Read the model definition and answer for the solid it produces. Units are mm, in the model's axes. A direction names the side the tool comes from. Round coordinates to 2 decimals unless told otherwise and drop trailing zeros. Write each loop counter-clockwise with the first axis right and the second up, starting at its lowest first coordinate (ties: lowest second). Pieces come first, ordered by that corner, then holes. Notation, with made-up numbers: (31.25, 35) - (79.25, 35) arc R16 ccw to (79.25, 66) - close; hole circle Ø11 at (59, 12.5). An arc over 180 degrees is marked (long way). Answer as CSV lines item,"result". Start each with the question number.
1) Consider line 1 along X through (y, z) = (11.5, 0); line 2 along X through (y, z) = (19, -8.5); line 3 along Z through (x, y) = (11.5, 35.5). Determine where each line is inside the solid, lowest interval first.
2) For a pull along Y with two mould halves and no side action, classify faces 1 (the cylindrical face through (19.54, 4.55, -19.7)), 2 (the cylindrical face through (15.747, 2.986, 8.191)), 3 (the flat face through (6.3, 0, 16)) as +Y half, -Y half, draft (parallel to the pull), parting line (faces both ways), or undercut.
3) Find section D-D on y = 19. Determine the outline of the cut face in (x, z).
4) Find section C-C on y = 3. Determine the outline of the cut face in (x, z), then the cut area to 3 significant figures.
5) Which of the six approach directions +Z, -Z, +X, -X, +Y, -Y give full straight-line access (tool end or side, diameter ignored) to faces 4 (the flat face through (0, 5, -23.5)), 5 (the cylindrical face through (-14.531, 0.507, -15.846)), 6 (the cylindrical face through (19.524, 24.224, -4.336))?
6) Each of these flat-tipped pins is pushed along its axis until it touches: pin 1 (10 mm diameter, centred on x = 1, y = 17.5, fed in from +Z); pin 2 (9 mm diameter, centred on x = 17.68, z = 17.68, fed in from +Y); pin 3 (12 mm diameter, centred on x = 10.5, y = 24, fed in from +Z). Where does it stop, or does it pass through?
from build123d import *

# Parameters (mm, degrees)
SKETCH_4_R           = 2.75
CUT_EXTRUDE_1_DEPTH  = 54.141321022
SKETCH_5_OUTSIDE_W   = 80.762
SKETCH_5_OUTSIDE_H   = 80.762
SKETCH_5_OUTSIDE_W_2 = 47
SKETCH_5_OUTSIDE_H_2 = 47
CUT_EXTRUDE_2_DEPTH  = 54.141321022


with BuildPart() as part:
    # Sketch 1 → Revolve 1 (revolve)
    with BuildSketch(Plane.XY, mode=Mode.PRIVATE) as revolve_1_sk:
        Polygon((-17, 0), (-21.5, 0), (-21.5, 1), (-30, 1), (-30, 8), (-20, 8), (-20, 40), (-17, 40), (-17, 38), (-17.75, 38), (-17.75, 36), (-17, 36), (-17, 4), (-17.75, 4), (-17.75, 2), (-17, 2), align=None)
    revolve(revolve_1_sk.sketch.rotate(Axis((0, 50.260536223, 0), (0, -1, 0)), 270), axis=Axis((0, 50.260536223, 0), (0, -1, 0)))

    # Sketch 4 → Cut-Extrude 1 (cut, through all)
    with BuildSketch(Plane(origin=(0, 8, 0), x_dir=(1, 0, 0), z_dir=(0, 1, 0))):
        with Locations(Location((-17.67766953, 17.67766953, 0), (0, 0, 270))):
            Circle(SKETCH_4_R)
        with Locations(Location((-17.67766953, -17.67766953, 0), (0, 0, 270))):
            Circle(SKETCH_4_R)
        with Locations(Location((17.67766953, 17.67766953, 0), (0, 0, 270))):
            Circle(SKETCH_4_R)
        with Locations(Location((17.67766953, -17.67766953, 0), (0, 0, 270))):
            Circle(SKETCH_4_R)
    extrude(amount=-CUT_EXTRUDE_1_DEPTH, mode=Mode.SUBTRACT)

    # Sketch 5 outside → Cut-Extrude 2 (cut, through all)
    with BuildSketch(Plane(origin=(0, 8, 0), x_dir=(1, 0, 0), z_dir=(0, 1, 0))):
        Rectangle(SKETCH_5_OUTSIDE_W, SKETCH_5_OUTSIDE_H)
        Rectangle(SKETCH_5_OUTSIDE_W_2, SKETCH_5_OUTSIDE_H_2, mode=Mode.SUBTRACT)
    extrude(amount=-CUT_EXTRUDE_2_DEPTH, mode=Mode.SUBTRACT)


solid = part.part
Check values:
1,line 1,"x = -20 to -17, 17 to 20"
1,line 2,"x = -18.1 to -14.72, 14.72 to 18.1"
1,line 3,"z = -16.36 to -12.52, 12.52 to 16.36"
2,face 1,"draft"
2,face 2,"undercut"
2,face 3,"-Y half"
3,outline,"circle Ø40 at (0, 0); hole circle Ø34 at (0, 0)"
4,outline,"(-23.5, -18.65) arc R30 ccw to (-18.65, -23.5) - (18.65, -23.5) arc R30 ccw to (23.5, -18.65) - (23.5, 18.65) arc R30 ccw to (18.65, 23.5) - (-18.65, 23.5) arc R30 ccw to (-23.5, 18.65) - close; hole circle Ø5.5 at (-17.68, -17.68); hole circle Ø5.5 at (-17.68, 17.68); hole circle Ø35.5 at (0, 0); hole circle Ø5.5 at (17.68, -17.68); hole circle Ø5.5 at (17.68, 17.68)"
4,area,"1,080 mm^2"
5,face 4,"-Z, +X, -X, +Y, -Y"
5,face 5,"-Y"
5,face 6,"+Y"
6,pin 1,"stops at z = 20"
6,pin 2,"stops at y = 8"
6,pin 3,"stops at z = 19.49"
